Verification items for the finished model (mm, model axes). A direction names the side the tool comes from. Round coordinates to 2 decimals unless told otherwise and drop trailing zeros. Write each loop counter-clockwise with the first axis right and the second up, starting at its lowest first coordinate (ties: lowest second). Pieces come first, ordered by that corner, then holes.
from build123d import *

# Parameters (mm, degrees)
F_1_4_20_TAPPED_HOLE1_D           = 5.1054
F_1_4_20_TAPPED_HOLE1_DEPTH       = 63.5
F_1_4_20_TAPPED_HOLE1_CSINK_D     = 7.62
F_1_4_20_TAPPED_HOLE1_CSINK_ANGLE = 90
F_1_4_20_TAPPED_HOLE1_TIP         = 1.533816902


with BuildPart() as part:
    # Sketch2 → Revolve1 (revolve)
    with BuildSketch(Plane.XY, mode=Mode.PRIVATE) as revolve1_sk:
        with BuildLine():
            Line((0, 121.620767237), (0, 6.473034307))
            Line((0, 6.473034307), (0, 1.393034307))
            Line((0, 1.393034307), (9.525, 1.393034307))
            Line((9.525, 1.393034307), (9.525, 6.473034307))
            Line((9.525, 6.473034307), (11.819732149, 6.473034307))
            Line((11.819732149, 6.473034307), (1.8977509, 119.881798927))
            ThreePointArc((1.8977509, 119.881798927), (1.286999346, 121.120280564), (0, 121.620767237))
        make_face()
    revolve(revolve1_sk.sketch.rotate(Axis((0, 6.473034307, 0), (0, 1, 0)), 90), axis=Axis((0, 6.473034307, 0), (0, 1, 0)))

    # 1/4-20 Tapped Hole1
    with Locations(Plane.XZ.offset(-1.393034307)):
        with Locations((0, 0)):
            CounterSinkHole(F_1_4_20_TAPPED_HOLE1_D / 2, F_1_4_20_TAPPED_HOLE1_CSINK_D / 2, depth=F_1_4_20_TAPPED_HOLE1_DEPTH, counter_sink_angle=F_1_4_20_TAPPED_HOLE1_CSINK_ANGLE)
            with Locations((0, 0, -(F_1_4_20_TAPPED_HOLE1_DEPTH + F_1_4_20_TAPPED_HOLE1_TIP / 2))):  # 118° drill point
                Cone(0, F_1_4_20_TAPPED_HOLE1_D / 2, F_1_4_20_TAPPED_HOLE1_TIP, mode=Mode.SUBTRACT)


solid = part.part
Q1. Material ranges on line 1 along X through (y, z) = (40, 0); line 2 along X through (y, z) = (19, 0); line 3 along X through (y, z) = (83, 1.5), recorded low to high.
Recorded:
line 1: x = -8.89 to -2.55, 2.55 to 8.89
line 2: x = -10.72 to -2.55, 2.55 to 10.72
line 3: x = -4.9 to 4.9
Q2. Depth check by flat-ended pin: P1, Ø12, axis at x = 1.5, y = 29, coming from the -Z side; P2, Ø1.5, axis at y = 35.5, z = 6.5, coming from the -X side; P3, Ø3, axis at x = -4.5, y = 39, coming from the -Z side. Enter the tip coordinate at first touch or a pass-through.
Recorded:
P1: stops at z = -10.36
P2: stops at x = -7.29
P3: stops at z = -8.48
Q3. Tool access check on faces 5 (the conical face through (-4.589, 63.971, 5.004)), 6 (the flat face through (-10, 6.473, 1)). Record the directions out of +Z, -Z, +X, -X, +Y, -Y that give a thin tool (end or side, any length) a straight path to the whole face; none if there is none.
Recorded:
face 5: +Y
face 6: -Y
Q4. Sectioned sample at A-A (y = 23). Enter the section's corners in (x, z), plus the area to 3 significant figures.
Recorded:
outline: circle Ø20.75 at (0, 0); hole circle Ø5.11 at (0, 0)
area: 318 mm2
Q5. Release check for a two-part mould opening along X. For faces 1 (the conical face through (0.423, 66.16, 0.133)), 2 (the flat face through (0, 1.393, 4)), 3 (the cylindrical face through (9.3, 3.97, 2.06)), 4 (the cylindrical face through (-2.435, 34.207, 0.767)) record: released by +X, released by -X, zero draft, split by the parting line, or undercut.
Recorded:
face 1: undercut
face 2: zero draft
face 3: split by the parting line
face 4: undercut
Q6. Sectioned sample at B-B (y = 46.5). Enter the section's corners in (x, z).
Recorded:
outline: circle Ø16.64 at (0, 0); hole circle Ø5.11 at (0, 0)
